from build123d import *

# Parameters (mm, degrees)
F0_R     = 7.14375
F1_DEPTH = 12.7


with BuildPart() as f1:
    # F0 (on Front) → F1 (new body)
    with BuildSketch(Plane.XZ):
        Polygon((120.559285, 134.108239), (-120.740715, 134.108239), (-120.740715, -65.916761), (6.259285, -65.916761), (6.259285, -15.116761), (120.559285, -15.116761), align=None)
        with Locations((-69.940715, 10.283239)):
            Circle(F0_R, mode=Mode.SUBTRACT)
        with Locations((63.409285, 10.283239)):
            Circle(F0_R, mode=Mode.SUBTRACT)
        with Locations((-69.940715, 96.008239)):
            Circle(F0_R, mode=Mode.SUBTRACT)
        with Locations((63.409285, 96.008239)):
            Circle(F0_R, mode=Mode.SUBTRACT)
    extrude(amount=F1_DEPTH)


solid = f1.part
Can you work these out from the model? Positions are in its coordinate system, mm. A direction names the side the tool comes from. Round coordinates to 2 decimals unless told otherwise and drop trailing zeros. Write each loop counter-clockwise with the first axis right and the second up, starting at its lowest first coordinate (ties: lowest second). Pieces come first, ordered by that corner, then holes. Notation, with made-up numbers: (57.25, -9.5) -> (92.25, -9.5) arc R15 ccw to (92.25, 19.5) -> close; hole circle Ø9 at (15, 75). An arc over 180 degrees is marked (long way). Use one line per item in the form item = value. Start each with the question number.
Q1. Which directions (+Z, -Z, +X, -X, +Y, -Y) give clear straight access to the entire face, cutting with the end or side of a thin tool? Please do faces 1 (the face through (-2, -12.7, 35)), 2 (the face through (63, -6, -15.117)).
Q2. Imagine slicing it at D-D (x = -66.5). Please give me the cut outline in (y, z).
Q3. If I drill on probe 1 along X at (y, z) = (-3.75, 100.5); probe 2 along Z at (x, y) = (-64, -1.5); probe 3 along X at (y, z) = (-7.5, 4.5), over which ranges is the centre line in solid material (lowest first)? Write a range as [from, to].
Q4. Imagine slicing it at A-A (y = -7.5). Please give me the cut outline in (x, z), then the cut area to 3 significant figures.
Q5. We'd pull the mould along X, two halves only. Please class faces 3 (the face through (57.74, -6.261, 5.936)), 4 (the face through (-120.741, -6, 35)), 5 (the face through (-2, 0, 35)), 6 (the face through (-71.49, -6.26, 3.31)): +X half, -X half, draft (parallel to the pull), parting line (faces both ways), or undercut.
Q6. Imagine slicing it at B-B (x = 66). Please give me the cut outline in (y, z).
Q7. I'm going to push a flat-ended pin straight in: P1, Ø2, axis at x = 41.5, y = -7, coming from the -Z side. Where does the tip first touch, or does it pass through?
Q8. Imagine slicing it at C-C (z = -51). Please give me the cut outline in (x, y), then the cut area to 3 significant figures.
Worked out:
q1.face_1 = +Z, -Z, +X, -X, -Y
q1.face_2 = -Z, +X, +Y, -Y
q2.outline = (-12.7, -65.92) -> (0, -65.92) -> (0, 4.02) -> (-12.7, 4.02) -> close; (-12.7, 16.54) -> (0, 16.54) -> (0, 89.75) -> (-12.7, 89.75) -> close; (-12.7, 102.27) -> (0, 102.27) -> (0, 134.11) -> (-12.7, 134.11) -> close
q3.probe_1 = [-120.74, -75.5], [-64.39, 57.85], [68.96, 120.56]
q3.probe_2 = [-65.92, 6.32], [14.25, 92.04], [99.98, 134.11]
q3.probe_3 = [-120.74, -74.13], [-65.75, 59.22], [67.6, 120.56]
q4.outline = (-120.74, -65.92) -> (6.26, -65.92) -> (6.26, -15.12) -> (120.56, -15.12) -> (120.56, 134.11) -> (-120.74, 134.11) -> close; hole circle Ø14.29 at (-69.94, 10.28); hole circle Ø14.29 at (-69.94, 96.01); hole circle Ø14.29 at (63.41, 10.28); hole circle Ø14.29 at (63.41, 96.01)
q4.area = 41,800 mm^2
q5.face_3 = undercut
q5.face_4 = -X half
q5.face_5 = draft
q5.face_6 = undercut
q6.outline = (-12.7, -15.12) -> (0, -15.12) -> (0, 3.63) -> (-12.7, 3.63) -> close; (-12.7, 16.94) -> (0, 16.94) -> (0, 89.35) -> (-12.7, 89.35) -> close; (-12.7, 102.67) -> (0, 102.67) -> (0, 134.11) -> (-12.7, 134.11) -> close
q7.P1 = -15.12
q8.outline = (-120.74, -12.7) -> (6.26, -12.7) -> (6.26, 0) -> (-120.74, 0) -> close
q8.area = 1,610 mm^2
